```python
from build123d import *

# Parameters (mm, degrees)
SKETCH1_R                   = 19
SKETCH1_R_2                 = 7
CONNECTOR_AXLE_SLEEVE_DEPTH = 59
SKETCH2_R                   = 31
SKETCH2_R_2                 = 11
OUTER_BOLT_FLANGE_DEPTH     = 19
SKETCH3_R                   = 26
SKETCH3_R_2                 = 9
STEPPED_HUB_SHOULDER_DEPTH  = 35
SKETCH4_R                   = 3.7
BOLT_CIRCLE_PAD_1_DEPTH     = 22
SKETCH5_R                   = 3.7
BOLT_CIRCLE_PAD_2_DEPTH     = 22
SKETCH6_R                   = 3.7
BOLT_CIRCLE_PAD_3_DEPTH     = 22
SKETCH7_R                   = 3.7
BOLT_CIRCLE_PAD_4_DEPTH     = 22
SKETCH8_R                   = 3.7
BOLT_CIRCLE_PAD_5_DEPTH     = 22
SKETCH9_R                   = 3.7
BOLT_CIRCLE_PAD_6_DEPTH     = 22


with BuildPart() as part:
    # Sketch1 → connector axle sleeve (new, symmetric)
    with BuildSketch(Plane(origin=(0, 0, 0), x_dir=(1, 0, 0), z_dir=(0, 1, 0))):
        with Locations(Location((0, 0, 0), (0, 0, 270))):
            Circle(SKETCH1_R)
        with Locations(Location((0, 0, 0), (0, 0, 270))):
            Circle(SKETCH1_R_2, mode=Mode.SUBTRACT)
    extrude(amount=CONNECTOR_AXLE_SLEEVE_DEPTH, both=True)

    # Sketch2 → outer bolt flange (add, symmetric)
    with BuildSketch(Plane(origin=(0, 0, 0), x_dir=(1, 0, 0), z_dir=(0, 1, 0))):
        with Locations(Location((0, 0, 0), (0, 0, 270))):
            Circle(SKETCH2_R)
        Circle(SKETCH2_R_2, mode=Mode.SUBTRACT)
    extrude(amount=OUTER_BOLT_FLANGE_DEPTH, both=True)

    # Sketch3 → stepped hub shoulder (add, symmetric)
    with BuildSketch(Plane(origin=(0, 0, 0), x_dir=(1, 0, 0), z_dir=(0, 1, 0))):
        with Locations(Location((0, 0, 0), (0, 0, 270))):
            Circle(SKETCH3_R)
        Circle(SKETCH3_R_2, mode=Mode.SUBTRACT)
    extrude(amount=STEPPED_HUB_SHOULDER_DEPTH, both=True)

    # Sketch4 → bolt circle pad 1 (add, symmetric)
    with BuildSketch(Plane(origin=(0, 0, 0), x_dir=(1, 0, 0), z_dir=(0, 1, 0))):
        with Locations((24, 0)):
            Circle(SKETCH4_R)
    extrude(amount=BOLT_CIRCLE_PAD_1_DEPTH, both=True)

    # Sketch5 → bolt circle pad 2 (add, symmetric)
    with BuildSketch(Plane(origin=(0, 0, 0), x_dir=(1, 0, 0), z_dir=(0, 1, 0))):
        with Locations((12, 20.784609691)):
            Circle(SKETCH5_R)
    extrude(amount=BOLT_CIRCLE_PAD_2_DEPTH, both=True)

    # Sketch6 → bolt circle pad 3 (add, symmetric)
    with BuildSketch(Plane(origin=(0, 0, 0), x_dir=(1, 0, 0), z_dir=(0, 1, 0))):
        with Locations((-12, 20.784609691)):
            Circle(SKETCH6_R)
    extrude(amount=BOLT_CIRCLE_PAD_3_DEPTH, both=True)

    # Sketch7 → bolt circle pad 4 (add, symmetric)
    with BuildSketch(Plane(origin=(0, 0, 0), x_dir=(1, 0, 0), z_dir=(0, 1, 0))):
        with Locations((-24, 0)):
            Circle(SKETCH7_R)
    extrude(amount=BOLT_CIRCLE_PAD_4_DEPTH, both=True)

    # Sketch8 → bolt circle pad 5 (add, symmetric)
    with BuildSketch(Plane(origin=(0, 0, 0), x_dir=(1, 0, 0), z_dir=(0, 1, 0))):
        with Locations((-12, -20.784609691)):
            Circle(SKETCH8_R)
    extrude(amount=BOLT_CIRCLE_PAD_5_DEPTH, both=True)

    # Sketch9 → bolt circle pad 6 (add, symmetric)
    with BuildSketch(Plane(origin=(0, 0, 0), x_dir=(1, 0, 0), z_dir=(0, 1, 0))):
        with Locations((12, -20.784609691)):
            Circle(SKETCH9_R)
    extrude(amount=BOLT_CIRCLE_PAD_6_DEPTH, both=True)


solid = part.part
```
Part model, mm, in its own coordinate system. A direction names the side the tool comes from. Give positions to 0.01 mm unless a question says otherwise; leave off trailing zeros. Write each loop counter-clockwise with the first axis right and the second up, starting at its lowest first coordinate (ties: lowest second). Pieces come first, ordered by that corner, then holes. Notation, with made-up numbers: (-3, 4.5) -> (13, 4.5) arc R15 cw to (13, 20.5) -> close; hole circle Ø7 at (14, 10). An arc over 180 degrees is marked (long way). Put each result on its own line as item: value. Start each with the question number.
Item 1: Pin check, flat tips, straight feed: pin 1 Ø2 at (x, z) = (-26.5, 0.5) entering from +Y; pin 2 Ø8 at (x, y) = (11.5, 0) entering from +Z; pin 3 Ø12 at (y, z) = (7.5, -23) entering from +X. Stop position of each tip, or through.
Item 2: Cut at C-C (y = -9). List the corners of the cut face in (x, z), then the cut area to 3 significant figures.
Item 3: Pull direction X, two halves, no side cores. Call faces 1 (the face through (-11.56, -46.83, -15.08)), 2 (the face through (0, 59, 8)), 3 (the face through (27.7, -20.5, 0.1)), 4 (the face through (-13.802, 20.521, -24.016)): pulls with the +X half, pulls with the -X half, needs draft (parallel to the pull), parting line crosses it, or undercut.
Item 4: Cut at D-D (z = 16.5). List the corners of the cut face in (x, y).
Item 5: Which spindle directions (+Z, -Z, +X, -X, +Y, -Y) get a long thin tool onto all of the face, cutting with end or side? Do faces 5 (the face through (13, 22, -23)), 6 (the face through (-11.56, 47.17, -15.08)), 7 (the face through (-14, 22, 23)), 8 (the face through (-21, -19, -16)), 9 (the face through (-14, -22, 23)). Say none if no direction does.
Item 6: Wall check: L1, parallel to X at y = -13, z = 0; L2, parallel to X at y = -29, z = 0; L3, parallel to Y at x = 21.5, z = 2. Give the ranges that are in metal, low to high. Write a range as [from, to].
Item 7: Cut at A-A (x = -3). List the corners of the cut face in (y, z).
Answer list:
1. pin 1: stops at y = 35
1. pin 2: stops at z = 30.08
1. pin 3: stops at x = 25.92
2. outline: circle Ø62 at (0, 0); hole circle Ø14 at (0, 0)
2. area: 2,870 mm2
3. face 1: parting line crosses it
3. face 2: needs draft
3. face 3: pulls with the +X half
3. face 4: undercut
4. outline: (-26.24, -19) -> (-20.09, -19) -> (-20.09, -35) -> (-9.42, -35) -> (-9.42, -59) -> (9.42, -59) -> (9.42, -35) -> (20.09, -35) -> (20.09, -19) -> (26.24, -19) -> (26.24, 19) -> (20.09, 19) -> (20.09, 35) -> (9.42, 35) -> (9.42, 59) -> (-9.42, 59) -> (-9.42, 35) -> (-20.09, 35) -> (-20.09, 19) -> (-26.24, 19) -> close
5. face 5: -Z, +X, +Y
5. face 6: +Y
5. face 7: +Z, -X, +Y
5. face 8: -Y
5. face 9: +Z, -X, -Y
6. L1: x = [-31, -7], [7, 31]
6. L2: x = [-26, -7], [7, 26]
6. L3: y = [-35, 35]
7. outline: (-59, -18.76) -> (-35, -18.76) -> (-35, -25.83) -> (-19, -25.83) -> (-19, -30.85) -> (19, -30.85) -> (19, -25.83) -> (35, -25.83) -> (35, -18.76) -> (59, -18.76) -> (59, -6.32) -> (-59, -6.32) -> close; (-59, 6.32) -> (59, 6.32) -> (59, 18.76) -> (35, 18.76) -> (35, 25.83) -> (19, 25.83) -> (19, 30.85) -> (-19, 30.85) -> (-19, 25.83) -> (-35, 25.83) -> (-35, 18.76) -> (-59, 18.76) -> close
